Here's how the part is built. I have some questions about the finished solid (model axes, mm). Face numbers are marked on the shaded views. A direction names the side the tool comes from. Coordinates: 2 decimals unless noted, no trailing zeros. Write each loop counter-clockwise with the first axis right and the second up, starting at its lowest first coordinate (ties: lowest second). Pieces come first, ordered by that corner, then holes.
from build123d import *

# Parameters (mm, degrees)
SKETCH_1_R      = 30
EXTRUDE_1_DEPTH = 8
FILLET_1_R      = 100
EXTRUDE_2_DEPTH = 10
FILLET_2_R      = 10
CHAMFER_1_SIZE  = 5


with BuildPart() as part:
    # 草图1 → 凸台-拉伸1 (new body)
    with BuildSketch(Plane.XY):
        Polygon((0, 0), (0, 280), (861.751390409, 0), align=None)
        with Locations((200, 100)):
            Circle(SKETCH_1_R, mode=Mode.SUBTRACT)
    extrude(amount=EXTRUDE_1_DEPTH)

    # 圆角1
    fillet_1_edges = [part.edges().sort_by_distance(p)[0] for p in [
        (861.751390409, 0, 4),
    ]]
    fillet(fillet_1_edges, radius=FILLET_1_R)

    # 草图2 → 凸台-拉伸2 (add)
    with BuildSketch(Plane.XY):
        with BuildLine():
            Line((0, 0), (230.376238942, 0))
            ThreePointArc((230.376238942, 0), (329.145073001, 84.356553496), (261.277938379, 195.10565163))
            Line((261.277938379, 195.10565163), (0, 280))
            Line((0, 280), (0, 0))
        make_face()
        Polygon((10, 266.236180795), (10, 35.358983849), (122.241374643, 229.766747442), align=None, mode=Mode.SUBTRACT)
        with BuildLine():
            Line((30, 10), (230.376238942, 10))
            ThreePointArc((230.376238942, 10), (319.268189595, 85.920898146), (258.187768435, 185.595086467))
            Line((258.187768435, 185.595086467), (151.410485182, 220.289128906))
            Line((151.410485182, 220.289128906), (30, 10))
        make_face(mode=Mode.SUBTRACT)
    extrude(amount=-EXTRUDE_2_DEPTH)

    # 圆角2
    fillet_2_edges = [part.edges().sort_by_distance(p)[0] for p in [
        (122.241374643, 229.766747442, -5),
        (10, 35.358983849, -5),
        (10, 266.236180795, -5),
        (151.410485182, 220.289128906, -5),
        (30, 10, -5),
    ]]
    fillet(fillet_2_edges, radius=FILLET_2_R)

    # 倒角1
    chamfer_1_edges = [part.edges().sort_by_distance(p)[0] for p in [
        (130.63896919, 237.552825815, 8),
        (329.145073001, 84.356553496, 8),
        (130.63896919, 237.552825815, -10),
        (329.145073001, 84.356553496, -10),
        (115.188119471, 0, -10),
        (115.188119471, 0, 8),
    ]]
    chamfer(chamfer_1_edges, length=CHAMFER_1_SIZE)


solid = part.part
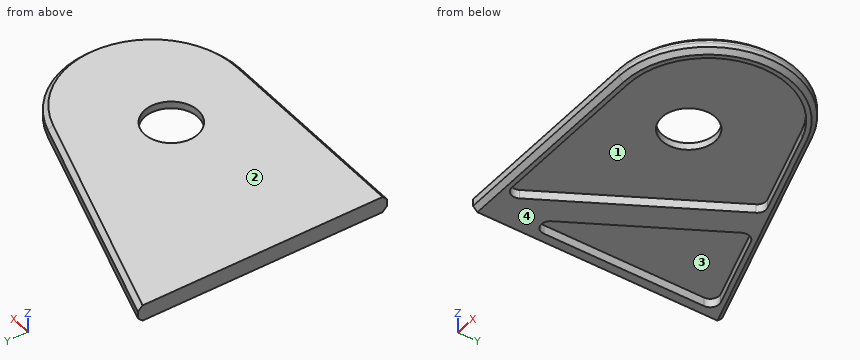
1. I want a section at C-C (y = 256.5). List the corners of the cut face in (x, z) for me.
2. I want a section at B-B (y = 100). List the corners of the cut face in (x, z) for me.
3. Thinking about a two-plate mould opening in X: for the marked faces 1 and 2, which applies, pulls with the +X half, pulls with the -X half, needs draft (parallel to the pull), parting line crosses it, or undercut?
4. For pin 1 Ø5 at (x, z) = (262.5, 1.5) entering from -Y; pin 2 Ø3 at (x, z) = (96, -6.5) entering from +Y; pin 3 Ø12 at (x, y) = (117.5, 36.5) entering from -Z, each with a flat end and sliding along its axis, tell me the tip position at first contact or that it passes through.
5. On a 3-axis mill with a long thin cutter (end or side, diameter ignored), from which of +Z, -Z, +X, -X, +Y, -Y can I reach the whole of each face in a straight line? I mean the marked faces 3 and 4. Say none if no direction works.
6. I want a section at A-A (x = 200). List the corners of the cut face in (y, z) for me, then the cut area to 3 significant figures.
7. If I drill on line 1 (X direction, y = 78, z = -4.5); line 2 (Y direction, x = 52, z = -1.25); line 3 (X direction, y = 120.5, z = -8), over which ranges is the centre line in solid material (lowest first)?
Response values:
1. outline: (0, -10) - (10.85, -10) - (10.85, 0) - (39.96, 0) - (39.96, -10) - (56.15, -10) - (72.33, -5) - (72.33, 3) - (56.15, 8) - (0, 8) - close
2. outline: (0, -10) - (10, -10) - (10, 0) - (47.32, 0) - (47.32, -10) - (81.96, -10) - (81.96, 0) - (170, 0) - (170, 8) - (0, 8) - close; (230, 0) - (320.38, 0) - (320.38, -10) - (325.38, -10) - (330.38, -5) - (330.38, 3) - (325.38, 8) - (230, 8) - close
3. face 1: undercut
3. face 2: needs draft
4. pin 1: stops at y = 4.49
4. pin 2: stops at y = 248.88
4. pin 3: stops at z = 0
5. face 3: -Z
5. face 4: -Z, +X, -X, +Y, -Y
6. outline: (0, -5) - (5, -10) - (10, -10) - (10, 0) - (70, 0) - (70, 8) - (5, 8) - (0, 3) - close; (130, 0) - (204.5, 0) - (204.5, -10) - (209.76, -10) - (215.02, -5) - (215.02, 3) - (209.76, 8) - (130, 8) - close
6. area: 1,390 mm2
7. line 1: x = 0 to 10, 34.62 to 69.26, 317.65 to 327.93
7. line 2: y = 0 to 10, 48.11 to 108.11, 252.59 to 263.1
7. line 3: x = 0 to 10, 59.16 to 93.8, 318.01 to 325.19
